Here's the drawing with two shaded views (mm, measured from the low corner). I have some questions. A direction names the side the tool comes from. Give positions to 0.01 mm unless a question says otherwise; leave off trailing zeros. Loops run counter-clockwise (first coordinate to the right, second up) from the corner with the lowest first, then second, coordinate; pieces in that order, holes last. Notation, with made-up numbers: M 61.5,26 L 71.5,26 A14 cw 71.5,47 Z; hole C -15.5,-22 d6. An arc over 180 degrees is marked long. Put each result on its own line as item: value. Start each with the question number.
1) Please list where these lines run through material, in increasing order: line 1 along X through (y, z) = (1.35, 9.75); line 2 along X through (y, z) = (1.2, 14.5) (1 decimal); line 3 along Y through (x, z) = (33.5, 11). Write a range as from..to.
2) Imagine slicing it at A-A (y = 1.7). Write out the boundary of the cut face in (x, z), then the cut area to 3 significant figures.
3) Imagine slicing it at D-D (x = 32.5). Write out the boundary of the cut face in (y, z).
4) If we mould it in two halves opening along X, with no side actions, what happens to the marked faces 1 and 2? For each: +X half, -X half, draft (parallel to the pull), parting line (faces both ways), or undercut.
5) For the marked faces 3 and 4, which set-ups out of +Z, -Z, +X, -X, +Y, -Y let a thin tool reach every point of the face, with its end or its side?
6) For P1, Ø1.5, axis at x = 28.5, y = 2.5, coming from the +Z side; P2, Ø8, axis at x = 31, z = 8, coming from the +Y side, each with a flat end and sliding along its axis, tell me the tip position at first contact or that it passes through.
7) Imagine slicing it at C-C (z = 1). Write out the boundary of the cut face in (x, y) (1 decimal), then the cut area to 3 significant figures.
8) Imagine slicing it at B-B (z = 12.75). Write out the boundary of the cut face in (x, y).
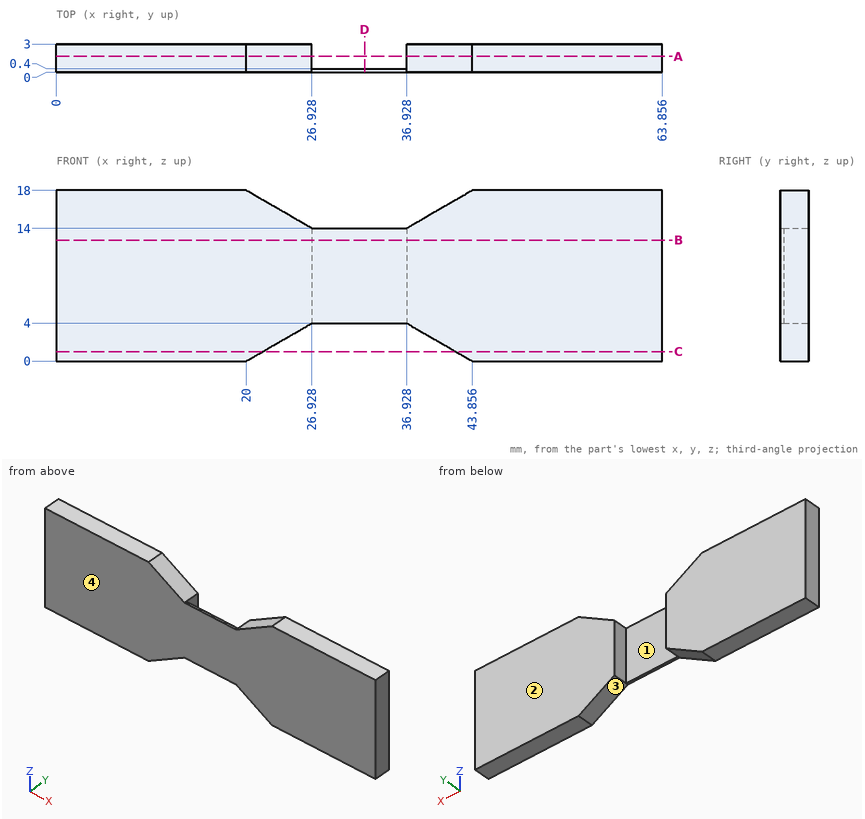
Recorded:
1. line 1: 0..26.93, 36.93..63.86
1. line 2: 0..26.1, 37.8..63.9
1. line 3: 0..0.4
2. outline: M 0,0 L 20,0 L 26.93,4 L 26.93,14 L 20,18 L 0,18 Z; M 36.93,4 L 43.86,0 L 63.86,0 L 63.86,18 L 43.86,18 L 36.93,14 Z
2. area: 914 mm²
3. outline: M 0,4 L 0.4,4 L 0.4,14 L 0,14 Z
4. face 1: undercut
4. face 2: draft
5. face 3: -Z, +Y, -Y
5. face 4: +Z, -Z, +X, -X, -Y
6. P1: through
6. P2: y = 0.4
7. outline: M 0,0 L 21.7,0 L 21.7,3 L 0,3 Z; M 42.1,0 L 63.9,0 L 63.9,3 L 42.1,3 Z
7. area: 130 mm²
8. outline: M 0,0 L 63.86,0 L 63.86,3 L 36.93,3 L 36.93,0.4 L 26.93,0.4 L 26.93,3 L 0,3 Z
